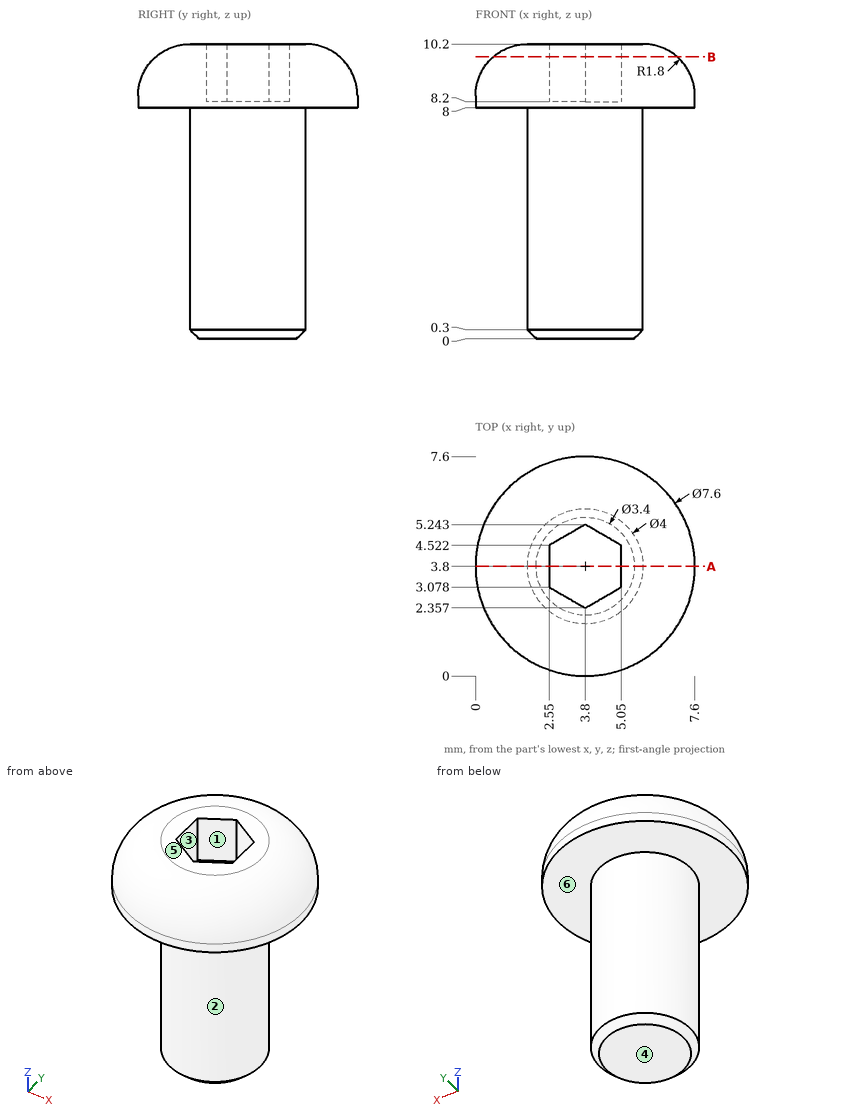
Check sheet for the drawn part. Datum: minimum x, y, z corner. Units: mm. A direction names the side the tool comes from. Coordinates: 2 decimals unless noted, no trailing zeros. Loops run counter-clockwise (first coordinate to the right, second up) from the corner with the lowest first, then second, coordinate; pieces in that order, holes last. Notation, with made-up numbers: (3, -32) -> (26, -32) arc R21 ccw to (26, -22) -> close; hole circle Ø11 at (43.5, 48.5). An arc over 180 degrees is marked (long way). Answer in a Markdown table with one row per item.
1. Go/stop test with flat-tipped pins: pin 1 (4 mm diameter, centred on x = 2.5, y = 6, fed in from -Z); pin 2 (4 mm diameter, centred on x = 5, z = 2, fed in from +Y); pin 3 (2 mm diameter, centred on x = 6.5, y = 6.5, fed in from -Z); pin 4 (1.2 mm diameter, centred on x = 3.5, y = 4, fed in from +Z). Record where each tip stops, or that it passes through.
Check values:
| item | result |
|---|---|
| pin 1 | stops at z = 0 |
| pin 2 | stops at y = 5.8 |
| pin 3 | stops at z = 8 |
| pin 4 | stops at z = 8.2 |
2. Release check for a two-part mould opening along Y. For the marked faces 1, 2, 3 and 4 record: released by +Y, released by -Y, zero draft, split by the parting line, or undercut.
Check values:
| item | result |
|---|---|
| face 1 | undercut |
| face 2 | split by the parting line |
| face 3 | undercut |
| face 4 | zero draft |
3. Material ranges on line 1 along Y through (x, z) = (2.75, 1.5); line 2 along Z through (x, y) = (1.75, 4); line 3 along Z through (x, y) = (3.25, 3.5), recorded low to high. Write a range as [from, to].
Check values:
| item | result |
|---|---|
| line 1 | y = [2.1, 5.5] |
| line 2 | z = [8, 10.2] |
| line 3 | z = [0, 8.2] |
4. Sectioned sample at B-B, the plane z = 9.75. Record the boundary of the cut face in (x, y).
Check values:
| item | result |
|---|---|
| outline | circle Ø6.38 at (3.8, 3.8); hole (2.55, 3.08) -> (3.8, 2.36) -> (5.05, 3.08) -> (5.05, 4.52) -> (3.8, 5.24) -> (2.55, 4.52) -> close |
5. Access from +Z, -Z, +X, -X, +Y, -Y to the whole of each face (thin tool, end or side, straight path). Record for the marked faces 5 and 6.
Check values:
| item | result |
|---|---|
| face 5 | +Z, +X, -X, +Y, -Y |
| face 6 | -Z |
6. Sectioned sample at A-A, the plane y = 3.8. Record the boundary of the cut face in (x, z).
Check values:
| item | result |
|---|---|
| outline | (0, 8) -> (1.8, 8) -> (1.8, 0.3) -> (2.1, 0) -> (5.5, 0) -> (5.8, 0.3) -> (5.8, 8) -> (7.6, 8) -> (7.6, 8.4) arc R1.8 ccw to (5.8, 10.2) -> (5.05, 10.2) -> (5.05, 8.2) -> (2.55, 8.2) -> (2.55, 10.2) -> (1.8, 10.2) arc R1.8 ccw to (0, 8.4) -> close |
